Could you check a few things on this drawing? It's one solid part, dimensions in mm from its lowest x, y, z. Give positions to 0.01 mm unless a question says otherwise; leave off trailing zeros. Loops run counter-clockwise (first coordinate to the right, second up) from the corner with the lowest first, then second, coordinate; pieces in that order, holes last. Notation, with made-up numbers: M 9,-1 L 63,-1 A23 ccw 63,22 Z; hole C -5,-33.5 d10. An arc over 180 degrees is marked long. Answer as CSV lines item,"result". Start each with the question number.
Item 1: I want a section at A-A on z = 27. List the corners of the cut face in (x, y) for me (3 decimals).
Item 2: Will these pins go through, and if not, where does the flat tip stop? P1, Ø2, axis at y = 59, z = 124.5, coming from the -X side; P2, Ø1, axis at x = 36.5, z = 59.5, coming from the +Y side (3 decimals); P3, Ø5, axis at y = 27, z = 101, coming from the +X side (3 decimals).
Item 3: If we mould it in two halves opening along Y, with no side actions, what happens to the marked faces 1, 2 and 3? For each: released by +Y, released by -Y, zero draft, split by the parting line, or undercut.
Item 4: If I drill on line 1 along X through (y, z) = (82, 148) (3 decimals), over which ranges is the centre line in solid material (lowest first)? Write a range as from..to.
Item 5: I want a section at B-B on x = 199. List the corners of the cut face in (y, z) for me (3 decimals), plus the area to 3 significant figures.
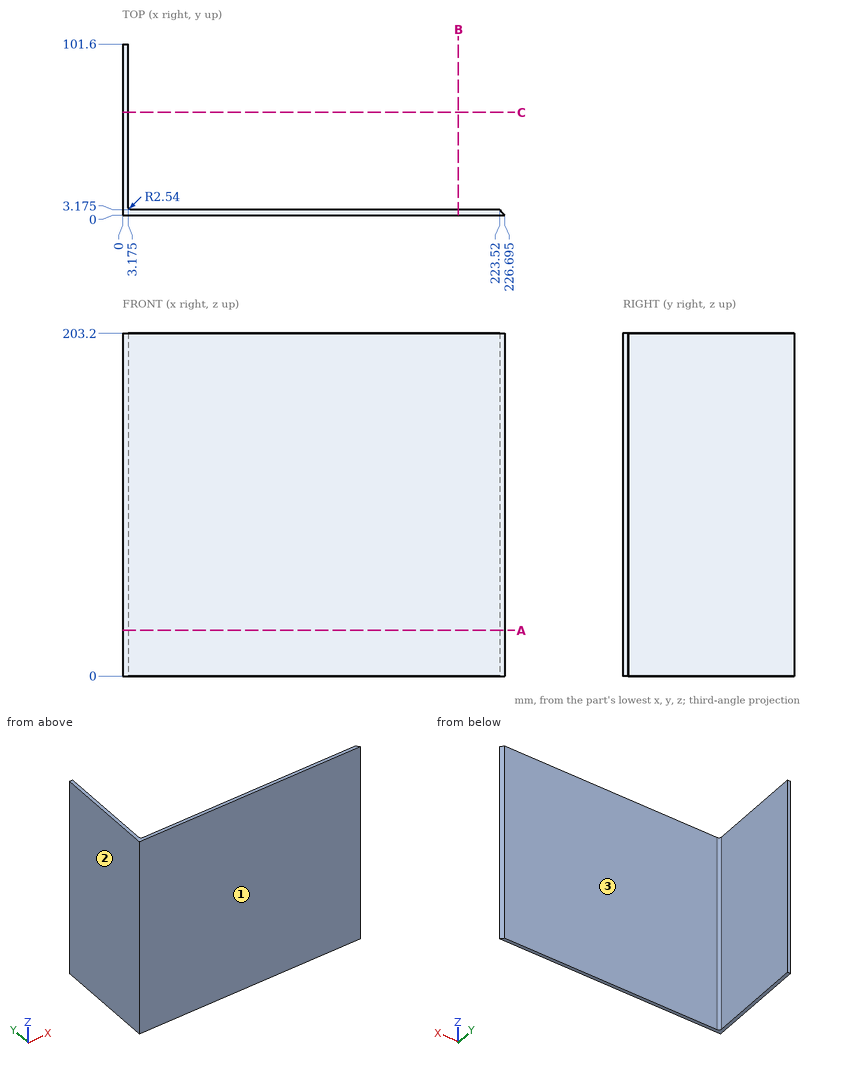
Result:
1,outline,"M 0,0 L 226.695,0 L 223.52,3.175 L 5.715,3.175 A2.54 cw 3.175,5.715 L 3.175,101.6 L 0,101.6 Z"
2,P1,"x = 0"
2,P2,"y = 3.175"
2,P3,"x = 3.175"
3,face 1,"released by -Y"
3,face 2,"zero draft"
3,face 3,"released by +Y"
4,line 1,"0..3.175"
5,outline,"M 0,0 L 3.175,0 L 3.175,203.2 L 0,203.2 Z"
5,area,"645 mm^2"
